Input: part model. Units: mm. Frame: model coordinates. A direction names the side the tool comes from. Give positions to 0.01 mm unless a question says otherwise; leave off trailing zeros. Write each loop counter-clockwise with the first axis right and the second up, starting at its lowest first coordinate (ties: lowest second). Pieces come first, ordered by that corner, then holes. Notation, with made-up numbers: (-10, 89.5) - (31, 89.5) arc R23 ccw to (31, 106.5) - close; hole circle Ø9 at (84.5, 1.25). An arc over 180 degrees is marked (long way). Use a Markdown table: item, result. Add a question column.
1. Pin query (flat end, axial travel): pin 1 (1.5 mm diameter, centred on y = 15.5, z = -14.5, fed in from -X); pin 2 (4 mm diameter, centred on y = 10.5, z = -22.5, fed in from -X); pin 3 (8 mm diameter, centred on y = 13.5, z = -53, fed in from -X). Return the tip coordinate at first contact, or that it passes through.
2. Section query B-B, the plane y = 13.5. Return loops of the section in (x, z).
3. Section query A-A, the plane x = 17. Return loops of the section in (y, z).
4. Set-up query: faces 1 (the cylindrical face through (-85.84, 1.48, 18.9)), 2 (the flat face through (-89.28, 17.4, 51.26)), 3 (the flat face through (96.92, 14.86, 55.02)). Return all of +Z, -Z, +X, -X, +Y, -Y with unobstructed straight access to the full face (end or side cutting, diameter ignored); none if empty.
5. Mould query, pull axis Z, two halves, no side actions, for faces 4 (the cylindrical face through (1.292, 6.504, -104.18)), 5 (the flat face through (1, 15, 109.394)), 6 (the cylindrical face through (61.385, 17.395, 102.439)), 7 (the flat face through (-90, 25, -58)). Classes: released by +Z, released by -Z, zero draft, split by the parting line, or undercut.
6. Section query C-C, the plane x = 43. Return loops of the section in (y, z), plus the area to 3 significant figures.
7. Material intervals for probe 1 along Z at (x, y) = (48, 12); probe 2 along Y at (x, z) = (-73, -47); probe 3 along X at (y, z) = (7, 76), sorted ascending.
```python
from build123d import *

# Parameters (mm, degrees)
SALIENTE_EXTRUIR2_DEPTH = 5
SALIENTE_EXTRUIR3_DEPTH = 20
REDONDEO2_R             = 5
REDONDEO3_R             = 5
CROQUIS4_R              = 60
CORTAR_EXTRUIR1_DEPTH   = 10
CROQUIS3_R              = 90
CORTAR_EXTRUIR2_DEPTH   = 3


with BuildPart() as part:
    # Croquis1 → Saliente-Extruir2 (new body)
    with BuildSketch(Plane(origin=(0, 0, 0), x_dir=(1, 0, 0), z_dir=(0, 1, 0))):
        with BuildLine():
            Line((-119.224191345, -9.394190445), (-67.262667118, -99.394190445))
            ThreePointArc((-67.262667118, -99.394190445), (-59.942159042, -106.71469852), (-49.942159042, -109.394190445))
            Line((-49.942159042, -109.394190445), (53.980889412, -109.394190445))
            ThreePointArc((53.980889412, -109.394190445), (63.980889412, -106.71469852), (71.301397487, -99.394190445))
            Line((71.301397487, -99.394190445), (123.262921714, -9.394190445))
            ThreePointArc((123.262921714, -9.394190445), (125.942413639, 0.605809555), (123.262921714, 10.605809555))
            Line((123.262921714, 10.605809555), (71.301397487, 100.605809555))
            ThreePointArc((71.301397487, 100.605809555), (63.980889412, 107.926317631), (53.980889412, 110.605809555))
            Line((53.980889412, 110.605809555), (-49.942159042, 110.605809555))
            ThreePointArc((-49.942159042, 110.605809555), (-59.942159042, 107.926317631), (-67.262667118, 100.605809555))
            Line((-67.262667118, 100.605809555), (-119.224191345, 10.605809555))
            ThreePointArc((-119.224191345, 10.605809555), (-121.90368327, 0.605809555), (-119.224191345, -9.394190445))
        make_face()
    extrude(amount=SALIENTE_EXTRUIR2_DEPTH)

    # Croquis2 → Saliente-Extruir3 (add)
    with BuildSketch(Plane(origin=(0, 5, 0), x_dir=(1, 0, 0), z_dir=(0, 1, 0))):
        with BuildLine():
            Line((-67.262667118, 100.605809555), (-119.224191345, 10.605809555))
            ThreePointArc((-119.224191345, 10.605809555), (-121.90368327, 0.605809555), (-119.224191345, -9.394190445))
            Line((-119.224191345, -9.394190445), (-67.262667118, -99.394190445))
            ThreePointArc((-67.262667118, -99.394190445), (-59.942159042, -106.71469852), (-49.942159042, -109.394190445))
            Line((-49.942159042, -109.394190445), (53.980889412, -109.394190445))
            ThreePointArc((53.980889412, -109.394190445), (63.980889412, -106.71469852), (71.301397487, -99.394190445))
            Line((71.301397487, -99.394190445), (123.262921714, -9.394190445))
            ThreePointArc((123.262921714, -9.394190445), (125.942413639, 0.605809555), (123.262921714, 10.605809555))
            Line((123.262921714, 10.605809555), (71.301397487, 100.605809555))
            ThreePointArc((71.301397487, 100.605809555), (63.980889412, 107.926317631), (53.980889412, 110.605809555))
            Line((53.980889412, 110.605809555), (-49.942159042, 110.605809555))
            ThreePointArc((-49.942159042, 110.605809555), (-59.942159042, 107.926317631), (-67.262667118, 100.605809555))
        make_face()
        with BuildLine():
            Line((-62.932540099, 98.105809555), (-114.894064326, 8.105809555))
            ThreePointArc((-114.894064326, 8.105809555), (-116.90368327, 0.605809555), (-114.894064326, -6.894190445))
            Line((-114.894064326, -6.894190445), (-62.932540099, -96.894190445))
            ThreePointArc((-62.932540099, -96.894190445), (-57.442159042, -102.384571501), (-49.942159042, -104.394190445))
            Line((-49.942159042, -104.394190445), (53.980889412, -104.394190445))
            ThreePointArc((53.980889412, -104.394190445), (61.480889412, -102.384571501), (66.971270468, -96.894190445))
            Line((66.971270468, -96.894190445), (118.932794695, -6.894190445))
            ThreePointArc((118.932794695, -6.894190445), (120.942413639, 0.605809555), (118.932794695, 8.105809555))
            Line((118.932794695, 8.105809555), (66.971270468, 98.105809555))
            ThreePointArc((66.971270468, 98.105809555), (61.480889412, 103.596190612), (53.980889412, 105.605809555))
            Line((53.980889412, 105.605809555), (-49.942159042, 105.605809555))
            ThreePointArc((-49.942159042, 105.605809555), (-57.442159042, 103.596190612), (-62.932540099, 98.105809555))
        make_face(mode=Mode.SUBTRACT)
    extrude(amount=SALIENTE_EXTRUIR3_DEPTH)

    # Redondeo2
    redondeo2_edges = [part.edges().sort_by_distance(p)[0] for p in [
        (2.019365185, 0, -110.605809555),
        (63.980889412, 0, -107.926317631),
        (97.282159601, 0, -55.605809555),
        (125.942413639, 0, -0.605809555),
        (97.282159601, 0, 54.394190445),
        (63.980889412, 0, 106.71469852),
        (2.019365185, 0, 109.394190445),
        (-59.942159042, 0, 106.71469852),
        (-93.243429232, 0, 54.394190445),
        (-121.90368327, 0, -0.605809555),
        (-93.243429232, 0, -55.605809555),
        (-59.942159042, 0, -107.926317631),
    ]]
    fillet(redondeo2_edges, radius=REDONDEO2_R)

    # Redondeo3
    redondeo3_edges = [part.edges().sort_by_distance(p)[0] for p in [
        (-57.442159042, 5, -103.596190612),
        (-88.913302213, 5, -53.105809555),
        (-116.90368327, 5, -0.605809555),
        (-88.913302213, 5, 51.894190445),
        (-57.442159042, 5, 102.384571501),
        (2.019365185, 5, 104.394190445),
        (61.480889412, 5, 102.384571501),
        (92.952032582, 5, 51.894190445),
        (120.942413639, 5, -0.605809555),
        (92.952032582, 5, -53.105809555),
        (61.480889412, 5, -103.596190612),
        (2.019365185, 5, -105.605809555),
    ]]
    fillet(redondeo3_edges, radius=REDONDEO3_R)

    # Croquis4 → Cortar-Extruir1 (cut)
    with BuildSketch(Plane(origin=(0, 0, 0), x_dir=(-1, 0, 0), z_dir=(0, -1, 0))):
        with Locations(Location((-2.019365185, 0.605809555, 0), (0, 0, 90))):
            Circle(CROQUIS4_R)
    extrude(amount=-CORTAR_EXTRUIR1_DEPTH, mode=Mode.SUBTRACT)

    # Croquis3 → Cortar-Extruir2 (cut)
    with BuildSketch(Plane.XZ):
        with Locations(Location((2.019365185, -0.605809555, 0), (0, 0, 270))):
            Circle(CROQUIS3_R)
    extrude(amount=-CORTAR_EXTRUIR2_DEPTH, mode=Mode.SUBTRACT)


solid = part.part
```
Result sheet:
| question | item | result |
|---|---|---|
| 1 | pin 1 | stops at x = -117.41 |
| 1 | pin 2 | stops at x = -113.51 |
| 1 | pin 3 | stops at x = -97.06 |
| 2 | outline | (-119.22, -10.61) - (-67.26, -100.61) arc R20 ccw to (-49.94, -110.61) - (53.98, -110.61) arc R20 ccw to (71.3, -100.61) - (123.26, -10.61) arc R20 ccw to (123.26, 9.39) - (71.3, 99.39) arc R20 ccw to (53.98, 109.39) - (-49.94, 109.39) arc R20 ccw to (-67.26, 99.39) - (-119.22, 9.39) arc R20 ccw to start; hole (-114.89, -8.11) - (-62.93, -98.11) arc R15 ccw to (-49.94, -105.61) - (53.98, -105.61) arc R15 ccw to (66.97, -98.11) - (118.93, -8.11) arc R15 ccw to (118.93, 6.89) - (66.97, 96.89) arc R15 ccw to (53.98, 104.39) - (-49.94, 104.39) arc R15 ccw to (-62.93, 96.89) - (-114.89, 6.89) arc R15 ccw to start |
| 3 | outline | (0, -105.61) arc R5 ccw to (5, -110.61) - (25, -110.61) - (25, -105.61) - (10, -105.61) arc R5 cw to (5, -100.61) - (5, -58.71) - (3, -58.71) - (3, -89.35) - (0, -89.35) - close; (0, 88.14) - (3, 88.14) - (3, 57.49) - (5, 57.49) - (5, 99.39) arc R5 cw to (10, 104.39) - (25, 104.39) - (25, 109.39) - (5, 109.39) arc R5 ccw to (0, 104.39) - close |
| 4 | face 1 | -Y |
| 4 | face 2 | +Y |
| 4 | face 3 | +Z, +X, +Y, -Y |
| 5 | face 4 | undercut |
| 5 | face 5 | released by +Z |
| 5 | face 6 | undercut |
| 5 | face 7 | zero draft |
| 6 | outline | (0, -105.61) arc R5 ccw to (5, -110.61) - (25, -110.61) - (25, -105.61) - (10, -105.61) arc R5 cw to (5, -100.61) - (5, -44.43) - (3, -44.43) - (3, -80.73) - (0, -80.73) - close; (0, 79.52) - (3, 79.52) - (3, 43.22) - (5, 43.22) - (5, 99.39) arc R5 cw to (10, 104.39) - (25, 104.39) - (25, 109.39) - (5, 109.39) arc R5 ccw to (0, 104.39) - close |
| 6 | area | 644 mm² |
| 7 | probe 1 | z = -110.61 to -105.61, 104.39 to 109.39 |
| 7 | probe 2 | y = 3 to 5 |
| 7 | probe 3 | x = -80.77 to -73.84, 77.88 to 84.81 |
